The figure shows three views and two pictorial views of one solid part (mm, origin at its lowest corner). Answer the questions. A direction names the side the tool comes from. Give positions to 0.01 mm unless a question says otherwise; leave off trailing zeros. Loops run counter-clockwise (first coordinate to the right, second up) from the corner with the lowest first, then second, coordinate; pieces in that order, holes last. Notation, with made-up numbers: M 39,-22 L 93,-22 A18 ccw 93,-12 Z; hole C 46,66 d6. An arc over 180 degrees is marked long. Answer as a JSON object with one key per item and string values. Group by question number.
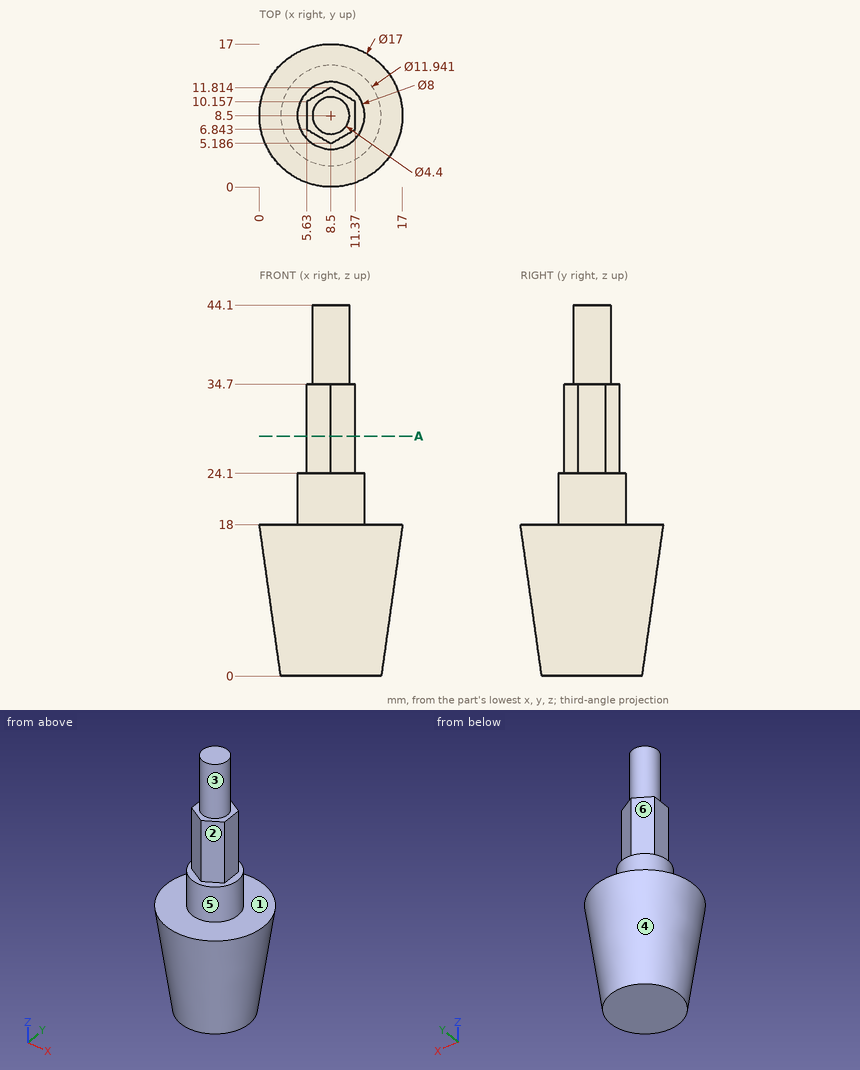
Item 1: Given pin 1 Ø2.5 at (y, z) = (8, 31.5) entering from -X; pin 2 Ø8 at (y, z) = (12.5, 33) entering from +X; pin 3 Ø1 at (x, z) = (4, 35) entering from +Y; pin 4 Ø1.5 at (x, y) = (4.5, 9.5) entering from +Z, each flat-ended and moving along its own axis, determine where each tip first touches the part or whether it passes through.
Item 2: For a pull along Y with two mould halves and no side action, classify the marked faces 1, 2 and 3 as pulls with the +Y half, pulls with the -Y half, needs draft (parallel to the pull), parting line crosses it, or undercut.
Item 3: Find the intervals of material crossed by probe 1 along Z at (x, y) = (9.25, 13); probe 2 along Z at (x, y) = (5.25, 7.5); probe 3 along X at (y, z) = (8.5, 24.5), in increasing order. Write a range as [from, to].
Item 4: A cutting plane is placed at A-A (z = 28.5). Determine the outline of the cut face in (x, y).
Item 5: A tool of negligible diameter and unlimited length cuts with its end or side. For the marked faces 4, 5 and 6, from which of +Z, -Z, +X, -X, +Y, -Y can it reach the whole face along a straight path? Write none if from no direction.
The answers:
{
 "1": {"pin 1": "stops at x = 5.63", "pin 2": "stops at x = 11.37", "pin 3": "passes through", "pin 4": "stops at z = 24.1"},
 "2": {"face 1": "needs draft", "face 2": "pulls with the -Y half", "face 3": "parting line crosses it"},
 "3": {"probe 1": "z = [0, 18]", "probe 2": "z = [0, 24.1]", "probe 3": "x = [5.63, 11.37]"},
 "4": {"outline": "M 5.63,6.84 L 8.5,5.19 L 11.37,6.84 L 11.37,10.16 L 8.5,11.81 L 5.63,10.16 Z"},
 "5": {"face 4": "-Z", "face 5": "+Z", "face 6": "+Z, -X, +Y"}
}
